The figure shows three views and two pictorial views of one solid part (mm, origin at its lowest corner). Answer the questions. A direction names the side the tool comes from. Round coordinates to 2 decimals unless told otherwise and drop trailing zeros. Order: outer loops, then holes, each group sorted by start corner. A loop starts at its lowest first (then second) coordinate and runs counter-clockwise, first axis right, second up. Notation, with made-up numbers: (5.25, 3) - (37.25, 3) arc R20 ccw to (37.25, 34) - close; hole circle Ø7 at (7, 37). An arc over 180 degrees is marked (long way). One line per item, written item: value. Start each with the question number.
1. Flat-ended cylindrical pins translate along their axes: P1, Ø2, axis at x = 146, y = 130, coming from the +Z side; P2, Ø1.5, axis at y = 107.5, z = 9, coming from the -X side; P3, Ø5.5, axis at x = 195.5, z = 15, coming from the +Y side; P4, Ø6, axis at y = 44, z = 13.5, coming from the -X side. Find the tip coordinate at first contact, or state that the pin passes through.
2. Section D-D, the plane x = 65.5 is taken. Give the vertices of the cut face in (y, z), then the cut area to 3 significant figures.
3. A tool of negligible diameter and unlimited length cuts with its end or side. For the marked faces 1, 2 and 3, from which of +Z, -Z, +X, -X, +Y, -Y can it reach the whole face along a straight path? Write none if from no direction.
4. Section B-B, the plane z = 15.5 is taken. Give the vertices of the cut face in (x, y) (1 decimal), then the cut area to 3 significant figures.
5. Section C-C, the plane y = 107.5 is taken. Give the vertices of the cut face in (x, z).
6. Section A-A, the plane z = 30.5 is taken. Give the vertices of the cut face in (x, y) (1 decimal), then the cut area to 3 significant figures.
7. Straight lines are drawn through the part: line 1 (Z direction, x = 34, y = 65); line 2 (Y direction, x = 89.5, z = 41); line 3 (X direction, y = 112, z = 25.5). For each, find the intervals that lie inside material, in ascending order.
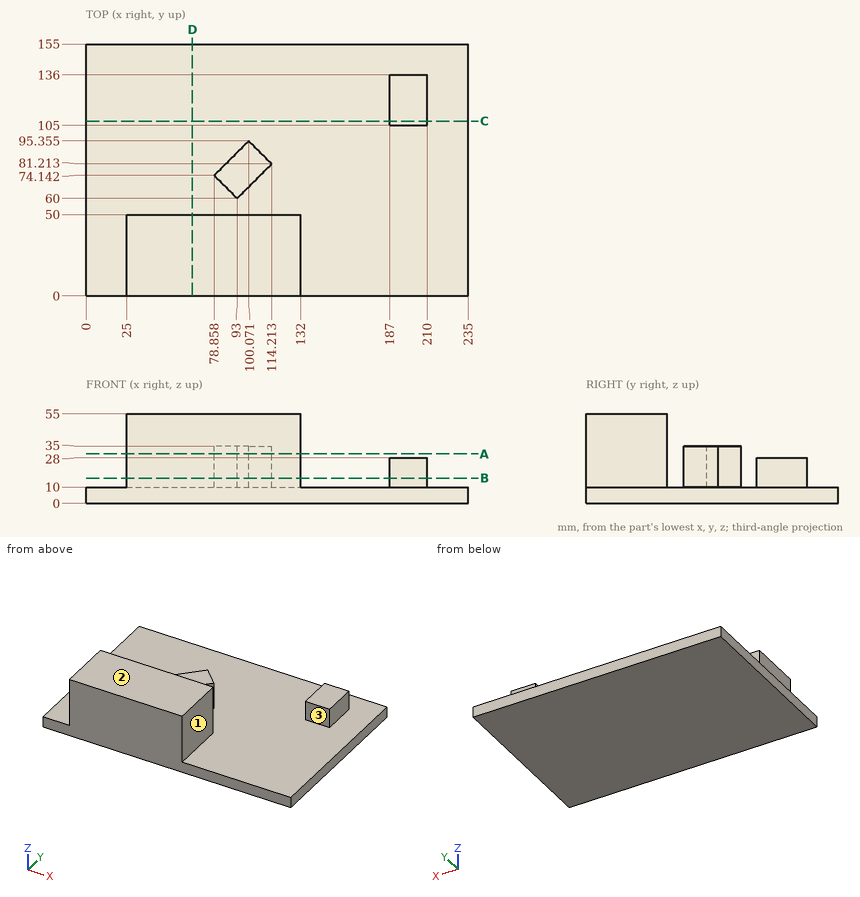
Answer list:
1. P1: stops at z = 10
1. P2: stops at x = 0
1. P3: stops at y = 136
1. P4: stops at x = 25
2. outline: (0, 0) - (155, 0) - (155, 10) - (50, 10) - (50, 55) - (0, 55) - close
2. area: 3,800 mm²
3. face 1: +Z, +X, +Y, -Y
3. face 2: +Z, +X, -X, +Y, -Y
3. face 3: +Z, +X, -X, -Y
4. outline: (25, 0) - (132, 0) - (132, 50) - (25, 50) - close; (78.9, 74.1) - (93, 60) - (114.2, 81.2) - (100.1, 95.4) - close; (187, 105) - (210, 105) - (210, 136) - (187, 136) - close
4. area: 6,660 mm²
5. outline: (0, 0) - (235, 0) - (235, 10) - (210, 10) - (210, 28) - (187, 28) - (187, 10) - (0, 10) - close
6. outline: (25, 0) - (132, 0) - (132, 50) - (25, 50) - close; (78.9, 74.1) - (93, 60) - (114.2, 81.2) - (100.1, 95.4) - close
6. area: 5,950 mm²
7. line 1: z = 0 to 10
7. line 2: y = 0 to 50
7. line 3: x = 187 to 210
